Part model, mm, in its own coordinate system. Face numbers are marked on the shaded views. A direction names the side the tool comes from. Round coordinates to 2 decimals unless told otherwise and drop trailing zeros. Loops run counter-clockwise (first coordinate to the right, second up) from the corner with the lowest first, then second, coordinate; pieces in that order, holes last. Notation, with made-up numbers: (49, 46) -> (86, 46) arc R12 ccw to (86, 50) -> close; hole circle Ø10 at (-23, -4.5). An arc over 180 degrees is marked (long way). Answer as CSV lines item,"result".
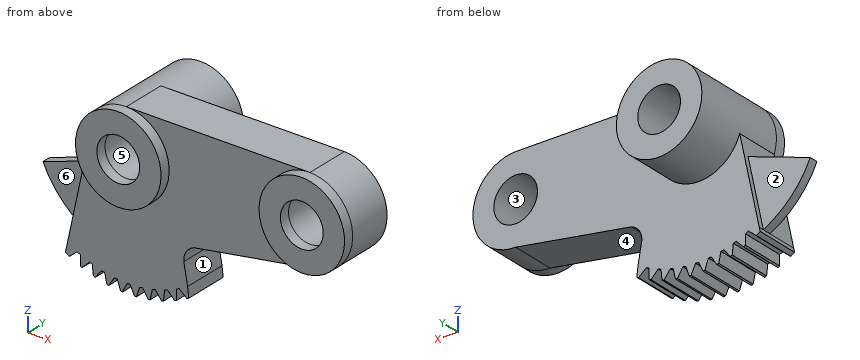
from build123d import *

# Parameters (mm, degrees)
SKETCH_1_R          = 2.5499999999999994
SKETCH_1_R_2        = 2.5499999999999976
EXTRUDE_1_DEPTH     = 5.1
SKETCH_2_R          = 4.999999999999998
SKETCH_2_R_2        = 2.5
EXTRUDE_2_DEPTH     = 5.94
CUT_EXTRUDE_1_DEPTH = 3.5
CUT_EXTRUDE_START   = -0.6
CUT_EXTRUDE_3_DEPTH = 0.6
EXTRUDE_START       = 1.2
SKETCH_6_R          = 4.999999999999998
SKETCH_6_R_2        = 2.5
SKETCH_6_R_3        = 5
SKETCH_6_R_4        = 2.4999999999999987
EXTRUDE_4_DEPTH     = 1.2


with BuildPart() as part:
    # Эскиз1 → Бобышка-Вытянуть1 (new body)
    with BuildSketch(Plane(origin=(0, 0, 0), x_dir=(1, 0, 0), z_dir=(0, 1, 0))):
        with BuildLine():
            Line((6.718023264525762, 8.928267668376021), (7.161238337218641, 11.37785065819786))
            Line((7.161238337218641, 11.37785065819786), (7.294846288705666, 12.560700282216452))
            Line((7.294846288705666, 12.560700282216452), (7.085001061393901, 12.665407082864023))
            Line((7.085001061393901, 12.665407082864023), (6.15987792536569, 11.916319971156167))
            Line((6.15987792536569, 11.916319971156167), (5.853623131200735, 12.10383694173367))
            Line((5.853623131200735, 12.10383694173367), (5.855060736117009, 13.29420757772634))
            Line((5.855060736117009, 13.29420757772634), (5.634886528714601, 13.37496556136943))
            Line((5.634886528714601, 13.37496556136943), (4.798663389284832, 12.527784837542624))
            Line((4.798663389284832, 12.527784837542624), (4.473480547373511, 12.680135526842204))
            Line((4.473480547373511, 12.680135526842204), (4.342730025112913, 13.863304415323501))
            Line((4.342730025112913, 13.863304415323501), (4.114949999467502, 13.919114749889351))
            Line((4.114949999467502, 13.919114749889351), (3.3779694438823102, 12.984318526945106))
            Line((3.3779694438823102, 12.984318526945106), (3.0378804853992434, 13.099618628946285))
            Line((3.0378804853992434, 13.099618628946285), (2.776558986480811, 14.260952083189514))
            Line((2.776558986480811, 14.260952083189514), (2.54399037483231, 14.291124494483034))
            Line((2.54399037483231, 14.291124494483034), (1.9153675367628848, 13.280274532718662))
            Line((1.9153675367628848, 13.280274532718662), (1.56457875493138, 13.35709799101592))
            Line((1.56457875493138, 13.35709799101592), (1.175918359734634, 14.482232389631033))
            Line((1.175918359734634, 14.482232389631033), (0.9414376205823001, 14.486393698794194))
            Line((0.9414376205823001, 14.486393698794194), (0.4289474421954887, 13.411992407470256))
            Line((0.42894744219548875, 13.411992407470256), (0.07179746795026506, 13.449389053044667))
            Line((0.07179746795026506, 13.449389053044667), (-0.4393947883485354, 14.524408492330128))
            Line((-0.43939478834853546, 14.524408492330128), (-0.6728875469021285, 14.502507231398162))
            Line((-0.6728875469021285, 14.502507231398162), (-1.062906477097084, 13.377843036257644))
            Line((-1.062906477097084, 13.377843036257644), (-1.4220003362283888, 13.375350339371238))
            Line((-1.4220003362283888, 13.375350339371238), (-2.049401918098927, 14.386958748197415))
            Line((-2.049401918098927, 14.386958748197415), (-2.279018807507275, 14.33926579666565))
            Line((-2.279018807507275, 14.33926579666565), (-2.5417426516817105, 13.178248785832608))
            Line((-2.5417426516817105, 13.178248785832608), (-2.898339045786024, 13.13589757669542))
            Line((-2.898339045786024, 13.13589757669542), (-3.6341901158202092, 14.071583165165732))
            Line((-3.6341901158202092, 14.071583165165732), (-3.8570911851181764, 13.998688399693854))
            Line((-3.8570911851181764, 13.998688399693854), (-3.989270518385492, 12.815678280718325))
            Line((-3.989270518385492, 12.815678280718325), (-4.3389589867331635, 12.733992368173748))
            Line((-4.3389589867331635, 12.733992368173748), (-5.174158380979493, 13.582182376127184))
            Line((-5.174158380979493, 13.582182376127184), (-5.3875867419063175, 13.48498737481814))
            Line((-5.3875867419063175, 13.48498737481814), (-5.3875867419063175, 12.2946158707315))
            Line((-5.3875867419063175, 12.2946158707315), (-5.751610974482103, 12.12883970299033))
            Line((-5.751610974482103, 12.12883970299033), (-6.666748566138722, 12.905854249247858))
            Line((-6.666748566138722, 12.905854249247858), (-7.13096440438616, 12.63943472468846))
            Line((-7.13096440438616, 12.63943472468846), (-7.025830916712447, 12.175864106991055))
            ThreePointArc((-7.025830916712449, 12.175864106991055), (-10.264322646127633, 9.799709596012173), (-12.51111253150909, 6.470163958468902))
            Line((-12.51111253150909, 6.470163958468902), (-5.241071220187256, 3.924995297345621))
            Line((-5.241071220187256, 3.924995297345621), (-4.737733567637334, 1.5980865565051285))
            ThreePointArc((-4.737733567637334, 1.5980865565051288), (-4.061430338102922, -2.9162962141622684), (1.55e-15, -5))
            Line((2.2e-16, -5), (21.46693589645179, -5.388260461869603))
            ThreePointArc((21.46693589645179, -5.388260461869605), (26.46693589645179, -0.3882604618696045), (21.46693589645179, 4.611739538130397))
            Line((21.46693589645179, 4.611739538130397), (7.924308406385933, 7.062073595968816))
            ThreePointArc((7.924308406385932, 7.062073595968816), (7.00463576208043, 7.790569444059032), (6.718023264525762, 8.928267668376021))
        make_face()
        with Locations(Location((21.46693589645179, -0.3882604618696021, 0), (0, 0, 270))):
            Circle(SKETCH_1_R, mode=Mode.SUBTRACT)
        with Locations(Location((2.78e-15, 1.83e-15, 0), (0, 0, 270))):
            Circle(SKETCH_1_R_2, mode=Mode.SUBTRACT)
    extrude(amount=EXTRUDE_1_DEPTH)

    # Эскиз2 → Бобышка-Вытянуть2 (add)
    with BuildSketch(Plane(origin=(0, 5.1, 0), x_dir=(1, 0, 0), z_dir=(0, 1, 0))):
        with Locations(Location((0, 0, 0), (0, 0, 270))):
            Circle(SKETCH_2_R)
        with Locations(Location((0, 0, 0), (0, 0, 270))):
            Circle(SKETCH_2_R_2, mode=Mode.SUBTRACT)
    extrude(amount=EXTRUDE_2_DEPTH)

    # Эскиз4 → Вырез-Вытянуть1 (cut)
    with BuildSketch(Plane.XZ):
        with BuildLine():
            Line((-5.241071220187255, -3.924995297345621), (-7.025830916712447, -12.175864106991055))
            ThreePointArc((-7.025830916712447, -12.175864106991055), (-10.264322646127628, -9.799709596012166), (-12.511112531509088, -6.470163958468901))
            Line((-12.511112531509088, -6.470163958468901), (-5.241071220187255, -3.924995297345621))
        make_face()
    extrude(amount=-CUT_EXTRUDE_1_DEPTH, mode=Mode.SUBTRACT)

    # Эскиз5 → Вырез-Вытянуть3 (cut)
    with BuildSketch(Plane(origin=(0, 5.1, 0), x_dir=(1, 0, 0), z_dir=(0, 1, 0)).offset(CUT_EXTRUDE_START)):
        with BuildLine():
            Line((-5.241071220187255, 3.924995297345621), (-7.025830916712447, 12.175864106991055))
            ThreePointArc((-7.025830916712447, 12.175864106991055), (-10.264322646127628, 9.799709596012168), (-12.511112531509088, 6.470163958468901))
            Line((-12.511112531509088, 6.470163958468901), (-5.241071220187255, 3.924995297345621))
        make_face()
    extrude(amount=CUT_EXTRUDE_3_DEPTH, mode=Mode.SUBTRACT)

    # Эскиз6 → Бобышка-Вытянуть4 (add)
    # profile 1 of 2: a face of its own
    with BuildSketch(Plane.XZ.offset(EXTRUDE_START)):
        with Locations(Location((0, 0, 0), (0, 0, 270))):
            Circle(SKETCH_6_R)
        with Locations(Location((0, 0, 0), (0, 0, 90))):
            Circle(SKETCH_6_R_2, mode=Mode.SUBTRACT)
    # profile 2 of 2: a face of its own
    with BuildSketch(Plane.XZ.offset(EXTRUDE_START)):
        with Locations(Location((21.46693589645179, 0.38826046186960295, 0), (0, 0, 270))):
            Circle(SKETCH_6_R_3)
        with Locations(Location((21.46693589645179, 0.38826046186960295, 0), (0, 0, 270))):
            Circle(SKETCH_6_R_4, mode=Mode.SUBTRACT)
    extrude(amount=-EXTRUDE_4_DEPTH)


solid = part.part
Q1. Saw through at D-D, the plane x = -9. Write the cut outline in (y, z).
Geometry results:
outline,"(3.5, -10.94) -> (4.5, -10.94) -> (4.5, -5.24) -> (3.5, -5.24) -> close"
Q2. Which spindle directions (+Z, -Z, +X, -X, +Y, -Y) get a long thin tool onto all of the face, cutting with end or side? Do the marked faces 4, 5 and 6. Say none if no direction does.
Geometry results:
face 4,"-Z, +X, +Y, -Y"
face 5,"none"
face 6,"+Z, -X, -Y"
Q3. Drill centre lines: line 1 along Y through (x, z) = (5.5, -0.75); line 2 along Z through (x, y) = (2, 6.5); line 3 along X through (y, z) = (8.3, 0). Where is each one in solid material? Low to high.
Geometry results:
line 1,"0 to 5.1"
line 2,"-4.58 to -1.5, 1.5 to 4.58"
line 3,"-5 to -2.5, 2.5 to 5"
Q4. Two-plate mould, pull along X, no slides. Class the marked faces 1, 2 and 3: pulls with the +X half, pulls with the -X half, needs draft (parallel to the pull), parting line crosses it, or undercut.
Geometry results:
face 1,"pulls with the +X half"
face 2,"needs draft"
face 3,"undercut"
Q5. Drop flat-ended pins along their axis: P1, Ø8, axis at x = 6, z = 1.5, coming from the -Y side; P2, Ø2.5, axis at x = 1, z = -0.5, coming from the +Y side; P3, Ø5, axis at x = -7, y = 8.5, coming from the -Z side; P4, Ø6, axis at x = 13.5, z = -1.5, coming from the -Y side. Give the stop position or say it passes through.
Geometry results:
P1,"y = -1.2"
P2,"through"
P3,"z = -2.18"
P4,"y = 0"
Q6. Saw through at B-B, the plane y = 2.5. Give the number of separate pieces and of enclosed holes in the cut face, then the cut area to 3 significant figures.
Geometry results:
separate pieces,"1"
enclosed holes,"2"
area,"387 mm2"
Q7. Saw through at C-C, the plane y = 9.25. Write the cut outline in (x, z).
Geometry results:
outline,"circle Ø10 at (0, 0); hole circle Ø5 at (0, 0)"
